Design review of the part built by this model. Coordinates are the model's own, in mm. A direction names the side the tool comes from. Coordinates: 2 decimals unless noted, no trailing zeros. Write each loop counter-clockwise with the first axis right and the second up, starting at its lowest first coordinate (ties: lowest second). Pieces come first, ordered by that corner, then holes. Notation, with made-up numbers: (16, 51) -> (72, 51) arc R26 ccw to (72, 78) -> close; hole circle Ø2 at (8.5, 13). An arc over 180 degrees is marked (long way). Write item = value, one per line. Start each with the question number.
Autodesk Fusion 360 part; units mm, degrees
sketch "Sketch1" plane through (0, 0, 0) normal (0, 0, 1) x (1, 0, 0) in component "Component"
  line L0 (3, 0) -> (12.8, 0)
  line L1 (15.8, 3) -> (15.8, 32.8)
  line L2 (12.8, 35.8) -> (3, 35.8)
  line L3 (0, 32.8) -> (0, 3)
  circle A0 centre (7.9, 28.5) radius 2.3
  line L4 (7.9, 35.8) -> (7.9, 0) construction
  line L5 (0, 17.9) -> (15.8, 17.9) construction
  circle A1 centre (7.9, 7.3) radius 2.3
  arc A2 (12.8, 0) -> (15.8, 3) centre (12.8, 3) ccw
  arc A3 (0, 3) -> (3, 0) centre (3, 3) ccw
  arc A4 (3, 35.8) -> (0, 32.8) centre (3, 32.8) ccw
  arc A5 (15.8, 32.8) -> (12.8, 35.8) centre (12.8, 32.8) ccw
  point P0 (15.8, 0)
  point P1 (0, 35.8)
  dimension "d1" = 15.8
  dimension "d2" = 35.8
  dimension "d3" = 4.6
  dimension "d4" = 7.3
  dimension "d5" = 3
extrude "Extrude1" add sketch "Sketch1" along normal blind 6.6 in component "Component"
sketch "Sketch2" plane through (0, 0, 6.6) normal (0, 0, 1) x (-1, 0, 0) in component "Component"
  circle A0 centre (-7.9, -28.5) radius 2.3
  circle A1 centre (-7.9, -7.3) radius 2.3
  arc A2 (-15.8, -32.8) -> (-12.8, -35.8) centre (-12.8, -32.8) ccw
  line L0 (-12.8, -35.8) -> (-3, -35.8)
  arc A3 (-3, -35.8) -> (0, -32.8) centre (-3, -32.8) ccw
  line L1 (0, -32.8) -> (0, -3)
  arc A4 (0, -3) -> (-3, 0) centre (-3, -3) ccw
  line L2 (-3, 0) -> (-12.8, 0)
  arc A5 (-12.8, 0) -> (-15.8, -3) centre (-12.8, -3) ccw
  line L3 (-15.8, -3) -> (-15.8, -32.8)
  circle A6 centre (-7.9, -28.5) radius 4.8
  circle A7 centre (-7.9, -7.3) radius 4.8
  dimension "d8" = 9.6
  dimension "d9" = 9.6
extrude "Extrude2" cut sketch "Sketch2" against normal blind 3.5 contours A6 | A7 in component "Component"
sketch "Sketch3" plane through (0, 0, 6.6) normal (0, 0, 1) x (-1, 0, 0) in component "Component"
  circle A0 centre (-7.9, -28.5) radius 4.8
  circle A1 centre (-7.9, -7.3) radius 4.8
  arc A2 (-15.8, -32.8) -> (-12.8, -35.8) centre (-12.8, -32.8) ccw
  line L0 (-12.8, -35.8) -> (-3, -35.8)
  arc A3 (-3, -35.8) -> (0, -32.8) centre (-3, -32.8) ccw
  line L1 (0, -32.8) -> (0, -3)
  arc A4 (0, -3) -> (-3, 0) centre (-3, -3) ccw
  line L2 (-3, 0) -> (-12.8, 0)
  arc A5 (-12.8, 0) -> (-15.8, -3) centre (-12.8, -3) ccw
  line L3 (-15.8, -3) -> (-15.8, -32.8)
  line L4 (0, -17.9) -> (-15.8, -17.9) construction
  circle A6 centre (-7.9, -17.9) radius 4.75
  dimension "d12" = 9.5
extrude "Extrude3" add sketch "Sketch3" along normal blind 6.6 contours A6 in component "Component"
ref_plane "WorkPlane2" through (7.9, 17.9, 3.3) normal (0, -1, 0) x (1, 0, 0) in component "Component"
sketch "Sketch6" plane through (7.9, 17.9, 3.3) normal (0, -1, 0) x (1, 0, 0) in component "Component"
  line L0 (4.75, 9.9) -> (-4.75, 9.9)
  line L1 (-4.75, 3.3) -> (4.75, 3.3)
  line L2 (-4.75, 3.3) -> (4.75, 3.3)
  line L3 (4.75, 3.3) -> (4.75, 7)
  line L4 (4.75, 7) -> (-4.75, 7)
  line L5 (-4.75, 7) -> (-4.75, 3.3)
  line L6 (0, 3.3) -> (0, 7) construction
  line L7 (1.8889, 7) -> (-1.8889, 7)
  line L8 (-1.8889, 7) -> (-1.8889, 3.3)
  line L9 (-1.8889, 3.3) -> (1.8889, 3.3)
  line L10 (1.8889, 3.3) -> (1.8889, 7)
  line L11 (1.8889, 7) -> (-1.8889, 3.3) construction
  line L12 (-1.8889, 7) -> (1.8889, 3.3) construction
  point P0 (0, 5.15)
  dimension "d19" = 3.7
  dimension "d20" = 3.7777
extrude "Extrude4" cut sketch "Sketch6" along normal through all and the other way through all contours L1 L2 L4 L5 L8 | L1 L2 L3 L4 L10 in component "Component"
sketch "Sketch7" plane through (0, 0, 13.2) normal (0, 0, 1) x (-1, 0, 0) in component "Component"
  circle A0 centre (-7.9, -17.9) radius 4.75
  line L0 (-13.2651, -15.3) -> (-2.5349, -15.3)
  line L1 (-2.5349, -15.3) -> (-2.5349, -20.5)
  line L2 (-2.5349, -20.5) -> (-13.2651, -20.5)
  line L3 (-13.2651, -20.5) -> (-13.2651, -15.3)
  line L4 (-13.2651, -15.3) -> (-2.5349, -20.5) construction
  line L5 (-2.5349, -15.3) -> (-13.2651, -20.5) construction
  point P0 (-7.9, -17.9)
  dimension "d22" = 5.2
ref_plane "WorkPlane3" through (7.9, 17.9, 3.3) normal (-1, 0, 0) x (0, -1, 0) in component "Component"
sketch "Sketch8" plane through (7.9, 17.9, 3.3) normal (-1, 0, 0) x (0, 1, 0) in component "Component"
  line L0 (-3.8726, -9.2) -> (3.2614, -9.2) construction
  line L1 (2.6, -9.9) -> (-2.6, -9.9)
  line L2 (0, -9.9) -> (0, -9.2) construction
  arc A0 (2.6, -9.9) -> (-2.6, -9.9) centre (0, -14.3786) ccw
  point P0 (-2.6, -9.9)
  point P1 (2.6, -9.9)
  dimension "d23" = 0.7
extrude "Extrude5" cut sketch "Sketch8" along normal through all and the other way through all in component "Component"
fillet "Fillet1" radius 1 8 edges at (7.9, 35.8, 6.6) (0.8787, 34.9213, 6.6) (0, 17.9, 6.6) (0.8787, 0.8787, 6.6) (7.9, 0, 6.6) (14.9213, 0.8787, 6.6) (15.8, 17.9, 6.6) (14.9213, 34.9213, 6.6) in component "Component"
fillet "Fillet1" radius 0.5 2 edges at (7.9, 13.15, 13.2) (7.9, 22.65, 13.2) in component "Component"
fillet "Fillet1" radius 0.5 2 edges at (12.65, 17.9, 12.5) (3.15, 17.9, 12.5) in component "Component"
component "Component" placed x (1, 0, 0) y (0, 1, 0) z (0, 0, 1) at (0, 0, 0)
equation "d4 = 5 mm + ( 4.6 / 2 ) * 1 mm"
equation "peg_diameter = 9.5 mm"
(1) Take a section at B-B, the plane x = 7.9. Count the separate pieces of the cut face and the enclosed holes in it, then the cut area to 3 significant figures.
(2) Mouldability with a two-part tool opening along Y and no side actions: class faces 4 (the face through (8.52, 23.74, 4.87)), 5 (the face through (14.9, 34.94, 2.76)), 6 (the face through (5, 18, 10.3)) as pulls with the +Y half, pulls with the -Y half, needs draft (parallel to the pull), parting line crosses it, or undercut.
(3) For line 1 (Y direction, x = 7.9, z = 2.25); line 2 (Y direction, x = 12.25, z = 5); line 3 (Z direction, x = 2, y = 4), list the stretches that pass through material, from the lowest coordinate up.
(4) For pin 1 Ø2 at (y, z) = (24, 2.5) entering from -X; pin 2 Ø1.1 at (y, z) = (16.5, 9.5) entering from -X; pin 3 Ø1.5 at (x, z) = (8, 8.5) entering from -Y; pin 4 Ø3 at (x, y) = (8.5, 26.5) entering from +Z, all flat-tipped, find the tip position at first contact; note any pin that passes through.
(5) Take a section at A-A, the plane y = 7.3. State the section outline as (x, z) points.
(6) For faces 1 (the face through (7, 5, 3.1)), 2 (the face through (14.94, 0.9, 2.76)), 3 (the face through (9.789, 18, 8)), list the 3-axis set-ups (+Z, -Z, +X, -X, +Y, -Y) from which the entire face can be reached by the end or side of a thin tool; tool diameter is ignored.
(7) Take a section at C-C, the plane z = 2. State the section outline as (x, y) points.
(8) Take a section at D-D, the plane y = 29. State the section outline as (x, z) points (3 decimals).
Report:
q1.separate_pieces = 3
q1.enclosed_holes = 0
q1.area = 200 mm2
q2.face_4 = undercut
q2.face_5 = pulls with the +Y half
q2.face_6 = needs draft
q3.line_1 = 0 to 5, 9.6 to 26.2, 30.8 to 35.8
q3.line_2 = 0 to 5.27, 9.33 to 26.47, 30.53 to 35.8
q3.line_3 = 0 to 6.6
q4.pin_1 = 0
q4.pin_2 = 6.01
q4.pin_3 = 13.15
q4.pin_4 = 3.1
q5.outline = (0, 0) -> (5.6, 0) -> (5.6, 3.1) -> (3.1, 3.1) -> (3.1, 6.6) -> (1, 6.6) arc R1 ccw to (0, 5.6) -> close; (10.2, 0) -> (15.8, 0) -> (15.8, 5.6) arc R1 ccw to (14.8, 6.6) -> (12.7, 6.6) -> (12.7, 3.1) -> (10.2, 3.1) -> close
q6.face_1 = +Z
q6.face_2 = +Z, -Z, +X, -Y
q6.face_3 = +X, +Y, -Y
q7.outline = (0, 3) arc R3 ccw to (3, 0) -> (12.8, 0) arc R3 ccw to (15.8, 3) -> (15.8, 32.8) arc R3 ccw to (12.8, 35.8) -> (3, 35.8) arc R3 ccw to (0, 32.8) -> close; hole circle Ø4.6 at (7.9, 7.3); hole circle Ø4.6 at (7.9, 28.5)
q8.outline = (0, 0) -> (5.655, 0) -> (5.655, 3.1) -> (3.126, 3.1) -> (3.126, 6.6) -> (1, 6.6) arc R1 ccw to (0, 5.6) -> close; (10.145, 0) -> (15.8, 0) -> (15.8, 5.6) arc R1 ccw to (14.8, 6.6) -> (12.674, 6.6) -> (12.674, 3.1) -> (10.145, 3.1) -> close
